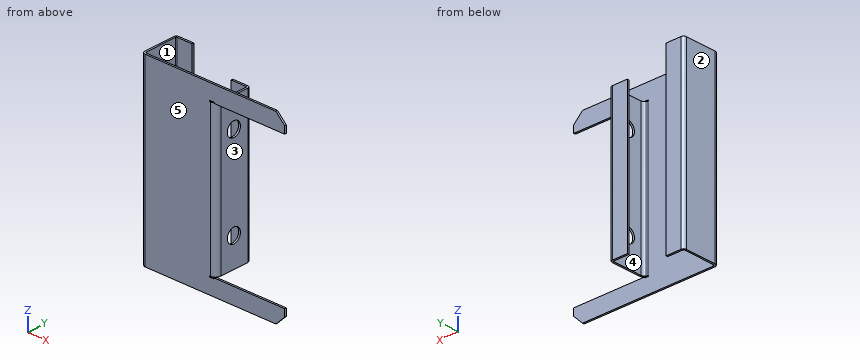
```python
from build123d import *

# Parameters (mm, degrees)
BASE_FLANGE1_DEPTH           = 1
BREAK_CORNER1_START          = 60.104076401
BREAK_CORNER1_OUTLINE_W      = 72.104076401
BREAK_CORNER1_OUTLINE_H      = 3
BREAK_CORNER1_DEPTH          = 3.535533906
BREAK_CORNER1_START_2        = -12
BREAK_CORNER1_2_OUTLINE_W    = 4.895923599
BREAK_CORNER1_2_OUTLINE_H    = 3
BREAK_CORNER1_2_DEPTH        = 11.292893219
EDGE_FLANGE1_STRIP_W         = 6
EDGE_FLANGE1_STRIP_H         = 1
EDGE_FLANGE1_STRIP_CUT_DEPTH = 100
EDGE_FLANGE1_DEPTH           = 100
EDGE_FLANGE2_STRIP_W         = 5
EDGE_FLANGE2_STRIP_H         = 1
EDGE_FLANGE2_STRIP_CUT_DEPTH = 100
EDGE_FLANGE2_DEPTH           = 100
EDGE_FLANGE3_START           = -2.5
EDGE_FLANGE3_OUTLINE_W       = 0.5
EDGE_FLANGE3_OUTLINE_H       = 1
EDGE_FLANGE3_DEPTH           = 2.5
EDGE_FLANGE3_START_2         = -1.23595
EDGE_FLANGE3_2_OUTLINE_W     = 19
EDGE_FLANGE3_2_OUTLINE_H     = 82
EDGE_FLANGE3_2_DEPTH         = 2.23595
EDGE_FLANGE3_3_OUTLINE_W     = 1
EDGE_FLANGE3_3_OUTLINE_H     = 82
EDGE_FLANGE3_3_DEPTH         = 0.70822
EDGE_FLANGE3_START_3         = -41
EDGE_FLANGE3_4_DEPTH         = 82
EDGE_FLANGE3_5_DEPTH         = 82
EDGE_FLANGE4_STRIP_W         = 5
EDGE_FLANGE4_STRIP_H         = 1
EDGE_FLANGE4_STRIP_CUT_DEPTH = 82
EDGE_FLANGE4_DEPTH           = 82
SKETCH18_R                   = 4
CUT_EXTRUDE1_DEPTH           = 10


with BuildPart() as part:
    # Base-Flange1: sheet metal written as solids
    # Sketch1 → Base-Flange1 (new body)
    with BuildSketch(Plane(origin=(0, 0, 0), x_dir=(1, 0, 0), z_dir=(0, 1, 0))):
        Polygon((39.172092849, 50), (40, 50), (40, 41), (0, 41), (0, -41), (40, -41), (40, -50), (-40, -50), (-40, 50), align=None)
    extrude(amount=-BASE_FLANGE1_DEPTH)

    # Break-Corner1: read off the stored shape, not the designer's step
    # Break-Corner1 outline → Break-Corner1 (cut)
    with BuildSketch(Plane(origin=(0, 0, 0), x_dir=(0.707106781186548, 0, -0.707106781186547), z_dir=(0.707106781186547, 0, 0.707106781186548)).offset(BREAK_CORNER1_START)):
        with Locations((24.052038201, -0.5)):
            Rectangle(BREAK_CORNER1_OUTLINE_W, BREAK_CORNER1_OUTLINE_H)
    extrude(amount=BREAK_CORNER1_DEPTH, mode=Mode.SUBTRACT)

    # Break-Corner1 2 outline → Break-Corner1 2 (cut)
    with BuildSketch(Plane(origin=(0, 0, 0), x_dir=(0.707106781186548, 0, -0.707106781186547), z_dir=(0.707106781186547, 0, 0.707106781186548)).offset(BREAK_CORNER1_START_2)):
        with Locations((62.552038201, -0.5)):
            Rectangle(BREAK_CORNER1_2_OUTLINE_W, BREAK_CORNER1_2_OUTLINE_H)
    extrude(amount=BREAK_CORNER1_2_DEPTH, mode=Mode.SUBTRACT)

    # Edge-Flange1: sheet metal written as solids
    # Edge-Flange1 strip (on a plane across the edge) → Edge-Flange1 strip cut (cut)
    with BuildSketch(Plane(origin=(-40, 0, -50), x_dir=(1, 0, 0), z_dir=(0, 0, 1))):
        with Locations((-2, -0.5)):
            Rectangle(EDGE_FLANGE1_STRIP_W, EDGE_FLANGE1_STRIP_H)
    extrude(amount=EDGE_FLANGE1_STRIP_CUT_DEPTH, mode=Mode.SUBTRACT)

    # Edge-Flange1 section (on a plane across the edge) → Edge-Flange1 (add)
    with BuildSketch(Plane(origin=(-40, 0, -50), x_dir=(1, 0, 0), z_dir=(0, 0, 1))):
        with BuildLine():
            Line((-1, 1), (-1, 19))
            Line((-1, 19), (0, 19))
            Line((0, 19), (0, 1))
            ThreePointArc((0, 1), (0.292893219, 0.292893219), (1, 0))
            Line((1, 0), (1, -1))
            ThreePointArc((1, -1), (-0.414213562, -0.414213562), (-1, 1))
        make_face()
    extrude(amount=EDGE_FLANGE1_DEPTH)

    # Edge-Flange2: sheet metal written as solids
    # Edge-Flange2 strip (on a plane across the edge) → Edge-Flange2 strip cut (cut)
    with BuildSketch(Plane(origin=(-40, 19, -50), x_dir=(0, -1, 0), z_dir=(0, 0, 1))):
        with Locations((-2, -0.5)):
            Rectangle(EDGE_FLANGE2_STRIP_W, EDGE_FLANGE2_STRIP_H)
    extrude(amount=EDGE_FLANGE2_STRIP_CUT_DEPTH, mode=Mode.SUBTRACT)

    # Edge-Flange2 section (on a plane across the edge) → Edge-Flange2 (add)
    with BuildSketch(Plane(origin=(-40, 19, -50), x_dir=(0, -1, 0), z_dir=(0, 0, 1))):
        with BuildLine():
            Line((-1, 0.5), (-1, 9))
            Line((-1, 9), (0, 9))
            Line((0, 9), (0, 0.5))
            ThreePointArc((0, 0.5), (0.146446609, 0.146446609), (0.5, 0))
            Line((0.5, 0), (0.5, -1))
            ThreePointArc((0.5, -1), (-0.560660172, -0.560660172), (-1, 0.5))
        make_face()
    extrude(amount=EDGE_FLANGE2_DEPTH)

    # Edge-Flange3: read off the stored shape, not the designer's step
    # Edge-Flange3 outline → Edge-Flange3 (cut)
    with BuildSketch(Plane(origin=(0, 0, 0), x_dir=(0, 0, -1), z_dir=(1, 0, 0)).offset(EDGE_FLANGE3_START)):
        with Locations((41.25, -0.5)):
            Rectangle(EDGE_FLANGE3_OUTLINE_W, EDGE_FLANGE3_OUTLINE_H)
        with Locations((-41.25, -0.5)):
            Rectangle(EDGE_FLANGE3_OUTLINE_W, EDGE_FLANGE3_OUTLINE_H)
    extrude(amount=EDGE_FLANGE3_DEPTH, mode=Mode.SUBTRACT)

    # Edge-Flange3 2 outline → Edge-Flange3 2 (add)
    with BuildSketch(Plane.YZ.offset(EDGE_FLANGE3_START_2)):
        with Locations((9.5, 0)):
            Rectangle(EDGE_FLANGE3_2_OUTLINE_W, EDGE_FLANGE3_2_OUTLINE_H)
    extrude(amount=EDGE_FLANGE3_2_DEPTH)

    # Edge-Flange3 3 outline → Edge-Flange3 3 (add)
    with BuildSketch(Plane.YZ):
        with Locations((-0.5, 0)):
            Rectangle(EDGE_FLANGE3_3_OUTLINE_W, EDGE_FLANGE3_3_OUTLINE_H)
    extrude(amount=EDGE_FLANGE3_3_DEPTH)

    # Edge-Flange3 4 outline → Edge-Flange3 4 (add)
    with BuildSketch(Plane.XY.offset(EDGE_FLANGE3_START_3)):
        with BuildLine():
            Line((-1.23595, -0.901073525), (-1.23595, 0.151696022))
            ThreePointArc((-1.23595, 0.151696022), (-1.610518266, 0.038290547), (-2, 0))
            Line((-2, 0), (-3, -1e-09))
            Line((-3, -1e-09), (-3, -0.999999999))
            Line((-3, -0.999999999), (-2, -1))
            ThreePointArc((-2, -1), (-1.614786147, -0.97516559), (-1.23595, -0.901073525))
        make_face()
    extrude(amount=EDGE_FLANGE3_4_DEPTH)

    # Edge-Flange3 5 outline → Edge-Flange3 5 (cut)
    with BuildSketch(Plane.XY.offset(EDGE_FLANGE3_START_3)):
        with BuildLine():
            Line((0, 2), (0, 19))
            Line((0, 19), (-1.23595, 19))
            Line((-1.23595, 19), (-1.23595, 0.151696022))
            ThreePointArc((-1.23595, 0.151696022), (-0.337456768, 0.888267119), (0, 2))
        make_face()
        with BuildLine():
            Line((1, 0), (1, 2))
            ThreePointArc((1, 2), (0.121320344, -0.121320344), (-2, -1))
            Line((-2, -1), (0.70822, -1))
            Line((0.70822, -1), (0.70822, 0))
            Line((0.70822, 0), (1, 0))
        make_face()
    extrude(amount=EDGE_FLANGE3_5_DEPTH, mode=Mode.SUBTRACT)

    # Edge-Flange4: sheet metal written as solids
    # Edge-Flange4 strip (on a plane across the edge) → Edge-Flange4 strip cut (cut)
    with BuildSketch(Plane(origin=(0, 19, 41), x_dir=(0, -1, 0), z_dir=(0, 0, -1))):
        with Locations((-2, -0.5)):
            Rectangle(EDGE_FLANGE4_STRIP_W, EDGE_FLANGE4_STRIP_H)
    extrude(amount=EDGE_FLANGE4_STRIP_CUT_DEPTH, mode=Mode.SUBTRACT)

    # Edge-Flange4 section (on a plane across the edge) → Edge-Flange4 (add)
    with BuildSketch(Plane(origin=(0, 19, 41), x_dir=(0, -1, 0), z_dir=(0, 0, -1))):
        with BuildLine():
            Line((-1, 0.5), (-1, 9))
            Line((-1, 9), (0, 9))
            Line((0, 9), (0, 0.5))
            ThreePointArc((0, 0.5), (0.146446609, 0.146446609), (0.5, 0))
            Line((0.5, 0), (0.5, -1))
            ThreePointArc((0.5, -1), (-0.560660172, -0.560660172), (-1, 0.5))
        make_face()
    extrude(amount=EDGE_FLANGE4_DEPTH)

    # Sketch18 → Cut-Extrude1 (cut)
    with BuildSketch(Plane(origin=(1, 0, 0), x_dir=(0, 0, -1), z_dir=(1, 0, 0))):
        with Locations(Location((-25, 10, 0), (0, 0, 90))):
            Circle(SKETCH18_R)
        with Locations(Location((25, 10, 0), (0, 0, 90))):
            Circle(SKETCH18_R)
    extrude(amount=-CUT_EXTRUDE1_DEPTH, mode=Mode.SUBTRACT)


solid = part.part
```
Check sheet for the modelled part. Datum: model origin and axes. Units: mm. Face numbers are marked on the shaded views. A direction names the side the tool comes from. Give positions to 0.01 mm unless a question says otherwise; leave off trailing zeros. Order: outer loops, then holes, each group sorted by start corner. A loop starts at its lowest first (then second) coordinate and runs counter-clockwise, first axis right, second up. Notation, with made-up numbers: M -16,54 L 41,54 A19 cw 41,62 Z; hole C 4,87 d10. An arc over 180 degrees is marked long. Answer in a Markdown table with one row per item. Add a question column.
Q1. Sectioned sample at B-B, the plane y = 10. Record the boundary of the cut face in (x, z).
Q2. Sectioned sample at C-C, the plane x = 23.5. Record the boundary of the cut face in (y, z).
Q3. Gauge pin test, flat ends, axial feed: pin 1 Ø0.5 at (y, z) = (19.5, 0) entering from -X; pin 2 Ø9 at (y, z) = (10.5, -4.5) entering from +X; pin 3 Ø1.1 at (y, z) = (19.5, 14.5) entering from +X; pin 4 Ø6 at (x, y) = (30, 1) entering from -Z. Record the tip position at first contact, or that the pin passes through.
Q4. Sectioned sample at D-D, the plane y = 4.5. Record the boundary of the cut face in (x, z).
Q5. Access from +Z, -Z, +X, -X, +Y, -Y to the whole of each face (thin tool, end or side, straight path). Record for the marked faces 1 and 2.
Q6. Sectioned sample at A-A, the plane z = -25. Record the boundary of the cut face in (x, y), and give its area (3 significant figures).
Q7. Thickness scan on L1, parallel to Z at x = 0.55, y = 10; L2, parallel to X at y = 16.25, z = 8.5; L3, parallel to Y at x = -9.5, z = -9. Record the ranges inside material, lowest first.
Q8. Release check for a two-part mould opening along X. For the marked faces 3, 4 and 5 record: released by +X, released by -X, zero draft, split by the parting line, or undercut.
Verdict:
| question | item | result |
|---|---|---|
| 1 | outline | M -41,-50 L -40,-50 L -40,50 L -41,50 Z; M 0,-41 L 1,-41 L 1,-29 L 0,-29 Z; M 0,-21 L 1,-21 L 1,21 L 0,21 Z; M 0,29 L 1,29 L 1,41 L 0,41 Z |
| 2 | outline | M -1,-50 L 0,-50 L 0,-41 L -1,-41 Z; M -1,41 L 0,41 L 0,50 L -1,50 Z |
| 3 | pin 1 | x = -40.8 |
| 3 | pin 2 | x = 1 |
| 3 | pin 3 | x = 0.93 |
| 3 | pin 4 | z = -50 |
| 4 | outline | M -41,-50 L -40,-50 L -40,50 L -41,50 Z; M 0,-41 L 1,-41 L 1,41 L 0,41 Z |
| 5 | face 1 | +Z, -Z |
| 5 | face 2 | +Z, -Z, -X, +Y, -Y |
| 6 | outline | M -41,1 A2 ccw -39,-1 L -2,-1 A3 ccw 1,2 L 1,6 L 0,6 L 0,2 A2 cw -2,0 L -39,0 A1 cw -40,1 L -40,18.5 A0.5 cw -39.5,19 L -31,19 L -31,20 L -39.5,20 A1.5 ccw -41,18.5 Z; M -9,19 L -0.5,19 A0.5 cw 0,18.5 L 0,14 L 1,14 L 1,18.5 A1.5 ccw -0.5,20 L -9,20 Z |
| 6 | area | 89.4 mm² |
| 7 | L1 | -41 to -29, -21 to 21, 29 to 41 |
| 7 | L2 | -41 to -40, 0 to 1 |
| 7 | L3 | -1 to 0 |
| 8 | face 3 | released by +X |
| 8 | face 4 | undercut |
| 8 | face 5 | zero draft |
